from build123d import *

# Parameters (mm, degrees)
SKETCH1_W           = 80
SKETCH1_H           = 10
BOSS_EXTRUDE1_DEPTH = 5
SKETCH2_W           = 10
SKETCH2_H           = 0.5
CUT_EXTRUDE1_DEPTH  = 81.777472107
SKETCH3_R           = 1.6
CUT_EXTRUDE2_DEPTH  = 81.777472107
SKETCH5_R           = 1.6
CUT_EXTRUDE3_DEPTH  = 81.777472107


with BuildPart() as part:
    # Sketch1 → Boss-Extrude1 (new, symmetric)
    with BuildSketch(Plane.XY):
        with Locations((40, 0)):
            Rectangle(SKETCH1_W, SKETCH1_H)
    extrude(amount=BOSS_EXTRUDE1_DEPTH, both=True)

    # Sketch2 → Cut-Extrude1 (cut, through all)
    with BuildSketch(Plane.XY.offset(5)):
        with Locations((5, 0)):
            Rectangle(SKETCH2_W, SKETCH2_H)
        with Locations((75, 0)):
            Rectangle(SKETCH2_W, SKETCH2_H)
    extrude(amount=-CUT_EXTRUDE1_DEPTH, mode=Mode.SUBTRACT)

    # Sketch3 → Cut-Extrude2 (cut, through all)
    with BuildSketch(Plane(origin=(0, 5, 0), x_dir=(1, 0, 0), z_dir=(0, 1, 0))):
        with Locations(Location((5, 0, 0), (0, 0, 180))):
            Circle(SKETCH3_R)
        with Locations(Location((75, 0, 0), (0, 0, 180))):
            Circle(SKETCH3_R)
    extrude(amount=-CUT_EXTRUDE2_DEPTH, mode=Mode.SUBTRACT)

    # Sketch5 → Cut-Extrude3 (cut, through all)
    with BuildSketch(Plane.XY.offset(5)):
        with Locations((15, 0)):
            Circle(SKETCH5_R)
        with Locations((65, 0)):
            Circle(SKETCH5_R)
    extrude(amount=-CUT_EXTRUDE3_DEPTH, mode=Mode.SUBTRACT)


solid = part.part
Read the model definition and answer for the solid it produces. Units are mm, in the model's axes. A direction names the side the tool comes from. Round coordinates to 2 decimals unless told otherwise and drop trailing zeros. Write each loop counter-clockwise with the first axis right and the second up, starting at its lowest first coordinate (ties: lowest second). Pieces come first, ordered by that corner, then holes.
1. The part is cut by section A-A, the plane z = 0. State how many separate pieces and enclosed holes the cut face has, then the cut area to 3 significant figures.
2. Which of the six approach directions +Z, -Z, +X, -X, +Y, -Y give full straight-line access (tool end or side, diameter ignored) to faces 5 (the face through (5, -0.25, 2)), 6 (the face through (73, -0.25, 0)), 7 (the face through (39, 0, 5))?
3. The part is cut by section B-B, the plane x = 65. Determine the outline of the cut face in (y, z), then the cut area to 3 significant figures.
4. Determine the mould class of faces 1 (the face through (80, -3, 0)), 2 (the face through (39, -5, 0)), 3 (the face through (39, 5, 0)), 4 (the face through (66.526, 0.481, 0.07)) for opening direction Y: pulls with the +Y half, pulls with the -Y half, needs draft (parallel to the pull), parting line crosses it, or undercut.
5. The part is cut by section D-D, the plane y = 3.5. Determine the outline of the cut face in (x, z), then the cut area to 3 significant figures.
6. Straight lines are drawn through the part: L1, parallel to X at y = 1, z = 0.5; L2, parallel to Y at x = 72, z = -1.75; L3, parallel to Z at x = 5, y = 3. For each, find the intervals that lie inside material, in ascending order.
7. The part is cut by section C-C, the plane x = 75. Determine the outline of the cut face in (y, z), then the cut area to 3 significant figures.
Values:
1. separate pieces: 5
1. enclosed holes: 2
1. area: 713 mm2
2. face 5: +Z, -Z, -X
2. face 6: +Z, -Z, +X
2. face 7: +Z, +X, -X, +Y, -Y
3. outline: (-5, -5) - (-1.6, -5) - (-1.6, 5) - (-5, 5) - close; (1.6, -5) - (5, -5) - (5, 5) - (1.6, 5) - close
3. area: 68.0 mm2
4. face 1: needs draft
4. face 2: pulls with the -Y half
4. face 3: pulls with the +Y half
4. face 4: undercut
5. outline: (0, -5) - (80, -5) - (80, 5) - (0, 5) - close; hole circle Ø3.2 at (5, 0); hole circle Ø3.2 at (75, 0)
5. area: 784 mm2
6. L1: x = 0 to 3.48, 6.52 to 13.75, 16.25 to 63.75, 66.25 to 73.48, 76.52 to 80
6. L2: y = -5 to -0.25, 0.25 to 5
6. L3: z = -5 to -1.6, 1.6 to 5
7. outline: (-5, -5) - (-0.25, -5) - (-0.25, -1.6) - (-5, -1.6) - close; (-5, 1.6) - (-0.25, 1.6) - (-0.25, 5) - (-5, 5) - close; (0.25, -5) - (5, -5) - (5, -1.6) - (0.25, -1.6) - close; (0.25, 1.6) - (5, 1.6) - (5, 5) - (0.25, 5) - close
7. area: 64.6 mm2
